Geometry: final body of the model. Coordinates: model frame, mm. Round coordinates to 2 decimals unless told otherwise and drop trailing zeros. Loops run counter-clockwise (first coordinate to the right, second up) from the corner with the lowest first, then second, coordinate; pieces in that order, holes last. Notation, with made-up numbers: (13, 30) -> (66, 30) arc R28 ccw to (66, 56) -> close; hole circle Ø7 at (-5.5, 67). An arc over 180 degrees is marked (long way). Answer in a Markdown table with one row per item.
```python
from build123d import *

# Parameters (mm, degrees)
F0_R     = 5.5
F0_R_2   = 4
F1_DEPTH = 10
F0_R_3   = 8
F2_DEPTH = 2


# Not quite as in the source:
# - a fillet or chamfer that OpenCascade refuses, or shapes differently, is made with other operations: its cross-section is extruded or revolved along the edge and cut away or added


with BuildPart() as f1:
    # F0 (on Top) → F1 (new body)
    with BuildSketch(Plane.XY):
        Circle(F0_R)
        Circle(F0_R_2, mode=Mode.SUBTRACT)
    extrude(amount=-F1_DEPTH)

    # F0 (on Top) → F2 (join)
    with BuildSketch(Plane.XY):
        Circle(F0_R_3)
        Circle(F0_R, mode=Mode.SUBTRACT)
        Circle(F0_R)
        Circle(F0_R_2, mode=Mode.SUBTRACT)
    extrude(amount=F2_DEPTH)

    # F3: fillet of radius 2 on 3 edges, made by hand

    # F3_s1 → F3_t2 (revolve, cut)
    with BuildSketch(Plane.XZ):
        with BuildLine():
            ThreePointArc((8, 0), (7.4142135624, 1.4142135624), (6, 2))
            Line((6, 2), (8, 2))
            Line((8, 2), (8, 0))
        make_face()
    revolve(axis=Axis((0, 0, 2), (0, 0, 1)), mode=Mode.SUBTRACT)

    # F3_s3 → F3_t4 (revolve, cut)
    with BuildSketch(Plane.XZ):
        with BuildLine():
            ThreePointArc((6, 2), (4.5857864376, 1.4142135624), (4, 0))
            Line((4, 0), (4, 2))
            Line((4, 2), (6, 2))
        make_face()
    revolve(axis=Axis((0, 0, 2), (0, 0, 1)), mode=Mode.SUBTRACT)

    # F3_s5 → F3_t6 (revolve, cut)
    with BuildSketch(Plane.XZ):
        with BuildLine():
            ThreePointArc((5.5, -8.0635083269), (5.0811388301, -9.2882531983), (4, -10))
            Line((4, -10), (5.5, -10))
            Line((5.5, -10), (5.5, -8.0635083269))
        make_face()
    revolve(axis=Axis((0, 0, -10), (0, 0, 1)), mode=Mode.SUBTRACT)


solid = f1.part
```
Item 1: Pin query (flat end, axial travel): pin 1 Ø4 at (y, z) = (1.5, 0.5) entering from -X; pin 2 Ø2 at (x, y) = (1, -3.5) entering from +Z; pin 3 Ø1.5 at (x, z) = (-5.5, -5.5) entering from -Y; pin 4 Ø1.5 at (x, z) = (-3.5, -6) entering from +Y. Return the tip coordinate at first contact, or that it passes through.
Answer:
| item | result |
|---|---|
| pin 1 | stops at x = -8 |
| pin 2 | stops at z = 1.47 |
| pin 3 | stops at y = -2.77 |
| pin 4 | stops at y = 4.76 |
Item 2: Line query: probe 1 along Y at (x, z) = (0, -4); probe 2 along X at (y, z) = (2.25, -8.5); probe 3 along X at (y, z) = (1.25, -8.5). Output: solid intervals per line, ascending. Write a range as [from, to].
Answer:
| item | result |
|---|---|
| probe 1 | y = [-5.5, -4], [4, 5.5] |
| probe 2 | x = [-4.97, -3.31], [3.31, 4.97] |
| probe 3 | x = [-5.31, -3.8], [3.8, 5.31] |
Item 3: Draft query along X for faces 1 (the face through (-1.19, -5.37, -3.98)), 2 (the face through (-0.867, -3.905, -5.07)), 3 (the face through (1.7, 5.4, 0)). Return one class per face: pulls with the +X half, pulls with the -X half, needs draft (parallel to the pull), parting line crosses it, or undercut.
Answer:
| item | result |
|---|---|
| face 1 | parting line crosses it |
| face 2 | undercut |
| face 3 | needs draft |
Item 4: Cut plane A-A (z = -0.25). Output: boundary loops of the cut face in (x, y).
Answer:
| item | result |
|---|---|
| outline | circle Ø11 at (0, 0); hole circle Ø8 at (0, 0) |
